Study the drawing (mm; zero at the part's minimum x, y, z) and answer. A direction names the side the tool comes from. Coordinates: 2 decimals unless noted, no trailing zeros. Order: outer loops, then holes, each group sorted by start corner. A loop starts at its lowest first (then second) coordinate and runs counter-clockwise, first axis right, second up.
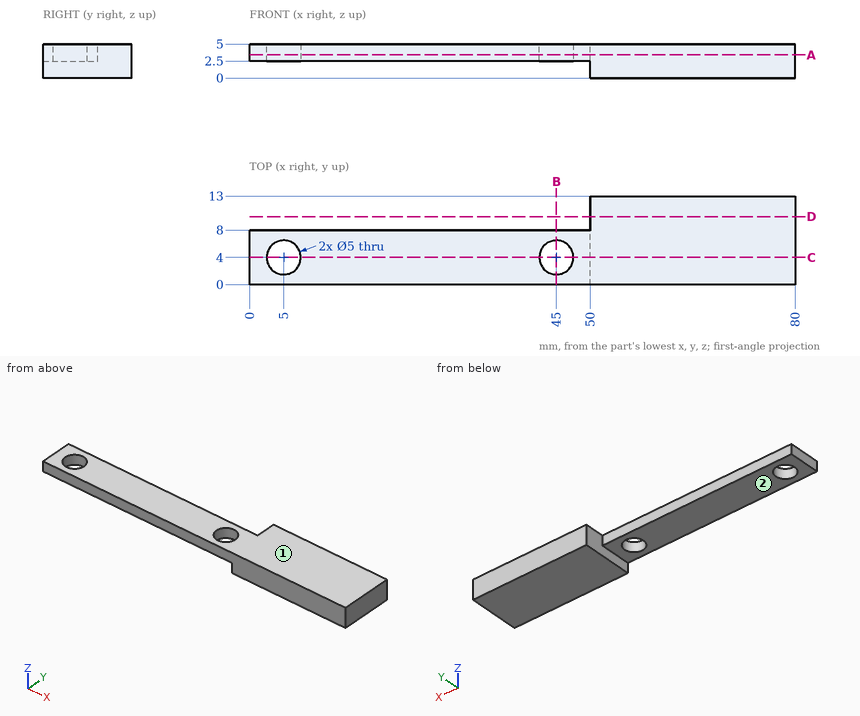
1) Which of the six approach directions +Z, -Z, +X, -X, +Y, -Y give full straight-line access (tool end or side, diameter ignored) to the marked faces 1 and 2?
A:
face 1: +Z, +X, -X, +Y, -Y
face 2: -Z, -X, +Y, -Y
2) A cutting plane is placed at A-A, the plane z = 3.4. Determine the outline of the cut face in (x, y), and give its area (3 significant figures).
A:
outline: (0, 0) - (80, 0) - (80, 13) - (50, 13) - (50, 8) - (0, 8) - close; hole circle Ø5 at (5, 4); hole circle Ø5 at (45, 4)
area: 751 mm2
3) A cutting plane is placed at C-C, the plane y = 4. Determine the outline of the cut face in (x, z).
A:
outline: (0, 2.5) - (2.5, 2.5) - (2.5, 5) - (0, 5) - close; (7.5, 2.5) - (42.5, 2.5) - (42.5, 5) - (7.5, 5) - close; (47.5, 2.5) - (50, 2.5) - (50, 0) - (80, 0) - (80, 5) - (47.5, 5) - close
4) Flat-ended cylindrical pins translate along their axes: pin 1 Ø0.8 at (x, z) = (29.5, 3.5) entering from +Y; pin 2 Ø6 at (x, y) = (9, 4.5) entering from -Z. Find the tip coordinate at first contact, or state that the pin passes through.
A:
pin 1: stops at y = 8
pin 2: stops at z = 2.5
5) A cutting plane is placed at B-B, the plane x = 45. Determine the outline of the cut face in (y, z).
A:
outline: (0, 2.5) - (1.5, 2.5) - (1.5, 5) - (0, 5) - close; (6.5, 2.5) - (8, 2.5) - (8, 5) - (6.5, 5) - close
6) Straight lines are drawn through the part: line 1 (X direction, y = 5.25, z = 2.55); line 2 (Y direction, x = 5, z = 3.85); line 3 (Y direction, x = 42, z = 2.9). For each, find the intervals that lie inside material, in ascending order.
A:
line 1: x = 0 to 2.83, 7.17 to 42.83, 47.17 to 80
line 2: y = 0 to 1.5, 6.5 to 8
line 3: y = 0 to 8
7) A cutting plane is placed at D-D, the plane y = 10. Determine the outline of the cut face in (x, z).
A:
outline: (50, 0) - (80, 0) - (80, 5) - (50, 5) - close
